Geometry: final body of the model. Coordinates: model frame, mm. Face numbers are marked on the shaded views. A direction names the side the tool comes from. Give positions to 0.01 mm unless a question says otherwise; leave off trailing zeros. Loops run counter-clockwise (first coordinate to the right, second up) from the corner with the lowest first, then second, coordinate; pieces in that order, holes last.
1. Section C-C, the plane y = 2.5. Output: boundary loops of the cut face in (x, z), then the cut area to 3 significant figures.
2. Section A-A, the plane y = -2. Output: boundary loops of the cut face in (x, z).
3. First-contact query: P1, Ø9, axis at x = -0.62, y = 5.58, coming from the -Z side; P2, Ø3, axis at x = -19, z = 0.5, coming from the +Y side; P3, Ø4, axis at x = -5, y = -2, coming from the +Z side; P4, Ø5, axis at x = -5, y = -2, coming from the -Z side. Flat tips, straight axial feed; report the tip coordinate or a pass-through.
4. Section D-D, the plane z = 3. Output: boundary loops of the cut face in (x, y) (3 decimals), then the cut area to 3 significant figures.
5. Draft query along Y for the marked faces 1, 2 and 3. Return one class per face: +Y half, -Y half, draft (parallel to the pull), parting line (faces both ways), or undercut.
6. Access query for the marked faces 4, 5 and 6. Directions: +Z, -Z, +X, -X, +Y, -Y. A direction counts if a zero-diameter tool reaches every point of the face in a straight line with its end or side. Return the directions, or none.
7. Section B-B, the plane z = -2. Output: boundary loops of the cut face in (x, y) (3 decimals), then the cut area to 3 significant figures.
8. Material intervals for line 1 along X through (y, z) = (-1, 0.5); line 2 along Y through (x, z) = (-5, 2.5); line 3 along Z through (x, y) = (0, -13.75), sorted ascending.
from build123d import *

# Parameters (mm, degrees)
SKETCH1_W                     = 46
SKETCH1_H                     = 36
BOSS_EXTRUDE1_DEPTH           = 8
M3X0_5_TAPPED_HOLE1_D         = 2.5
M3X0_5_TAPPED_HOLE1_DEPTH     = 7.5
M3X0_5_TAPPED_HOLE1_TIP       = 0.751075774
M3X0_5_TAPPED_HOLE2_D         = 2.5
M3X0_5_TAPPED_HOLE2_DEPTH     = 7.5
M3X0_5_TAPPED_HOLE2_TIP       = 0.751075774
FILLET2_R                     = 8
SKETCH13_W                    = 5
SKETCH13_H                    = 5
CUT_EXTRUDE1_DEPTH            = 4.5
CSK_FOR_M3_SFHCS1_D           = 3
CSK_FOR_M3_SFHCS1_DEPTH       = 9.5
CSK_FOR_M3_SFHCS1_CSINK_D     = 5.3
CSK_FOR_M3_SFHCS1_CSINK_ANGLE = 60
CSK_FOR_M3_SFHCS1_TIP         = 0.901290929
FILLET3_R                     = 1
HOLE1_D                       = 10
HOLE1_CBORE_D                 = 12
HOLE1_CBORE_DEPTH             = 3.3
CSK_FOR_M3_SFHCS2_D           = 3
CSK_FOR_M3_SFHCS2_DEPTH       = 9.5
CSK_FOR_M3_SFHCS2_CSINK_D     = 5.4
CSK_FOR_M3_SFHCS2_CSINK_ANGLE = 60
CSK_FOR_M3_SFHCS2_TIP         = 0.901290929


with BuildPart() as part:
    # Sketch1 → Boss-Extrude1 (new body)
    with BuildSketch(Plane.XY.offset(4.5)):
        Rectangle(SKETCH1_W, SKETCH1_H)
    extrude(amount=-BOSS_EXTRUDE1_DEPTH)

    # M3x0.5 Tapped Hole1
    with Locations(Plane(origin=(0, -18, 0), x_dir=(-1, 0, 0), z_dir=(0, -1, 0))):
        with Locations((0, -0.5)):
            Hole(M3X0_5_TAPPED_HOLE1_D / 2, depth=M3X0_5_TAPPED_HOLE1_DEPTH)
            with Locations((0, 0, -(M3X0_5_TAPPED_HOLE1_DEPTH + M3X0_5_TAPPED_HOLE1_TIP / 2))):  # 118° drill point
                Cone(0, M3X0_5_TAPPED_HOLE1_D / 2, M3X0_5_TAPPED_HOLE1_TIP, mode=Mode.SUBTRACT)

    # M3x0.5 Tapped Hole2
    with Locations(Plane(origin=(0, -18, 0), x_dir=(-1, 0, 0), z_dir=(0, -1, 0))):
        with Locations((-19, -0.5), (19, -0.5)):
            Hole(M3X0_5_TAPPED_HOLE2_D / 2, depth=M3X0_5_TAPPED_HOLE2_DEPTH)
            with Locations((0, 0, -(M3X0_5_TAPPED_HOLE2_DEPTH + M3X0_5_TAPPED_HOLE2_TIP / 2))):  # 118° drill point
                Cone(0, M3X0_5_TAPPED_HOLE2_D / 2, M3X0_5_TAPPED_HOLE2_TIP, mode=Mode.SUBTRACT)

    # Fillet2
    fillet2_edges = [part.edges().sort_by_distance(p)[0] for p in [
        (-23, 18, 0.5),
        (23, 18, 0.5),
    ]]
    fillet(fillet2_edges, radius=FILLET2_R)

    # Sketch13 → Cut-Extrude1 (cut)
    with BuildSketch(Plane.XY.offset(4.5)):
        with Locations((-5, -2)):
            Rectangle(SKETCH13_W, SKETCH13_H)
    extrude(amount=-CUT_EXTRUDE1_DEPTH, mode=Mode.SUBTRACT)

    # CSK for M3 SFHCS1
    with Locations(Plane(origin=(-5, -2, -3.5), x_dir=(-1, 0, 0), z_dir=(0, 0, -1))):
        with Locations((0, 0)):
            CounterSinkHole(CSK_FOR_M3_SFHCS1_D / 2, CSK_FOR_M3_SFHCS1_CSINK_D / 2, depth=CSK_FOR_M3_SFHCS1_DEPTH, counter_sink_angle=CSK_FOR_M3_SFHCS1_CSINK_ANGLE)
            with Locations((0, 0, -(CSK_FOR_M3_SFHCS1_DEPTH + CSK_FOR_M3_SFHCS1_TIP / 2))):  # 118° drill point
                Cone(0, CSK_FOR_M3_SFHCS1_D / 2, CSK_FOR_M3_SFHCS1_TIP, mode=Mode.SUBTRACT)

    # Fillet3
    fillet3_edges = [part.edges().sort_by_distance(p)[0] for p in [
        (-2.5, 0.5, 2.25),
        (-2.5, -4.5, 2.25),
        (-7.5, -4.5, 2.25),
        (-7.5, 0.5, 2.25),
    ]]
    fillet(fillet3_edges, radius=FILLET3_R)

    # Hole1 (through all)
    with Locations(Plane(origin=(0, 0, -3.5), x_dir=(-1, 0, 0), z_dir=(0, 0, -1))):
        with Locations((0.625, 5.577722283)):
            CounterBoreHole(HOLE1_D / 2, HOLE1_CBORE_D / 2, HOLE1_CBORE_DEPTH)

    # CSK for M3 SFHCS2
    with Locations(Plane.XY.offset(4.5)):
        with Locations((-10.337423522, 10.741909474), (8.703529058, 11.40683419), (-0.241105536, -5.415576815)):
            CounterSinkHole(CSK_FOR_M3_SFHCS2_D / 2, CSK_FOR_M3_SFHCS2_CSINK_D / 2, depth=CSK_FOR_M3_SFHCS2_DEPTH, counter_sink_angle=CSK_FOR_M3_SFHCS2_CSINK_ANGLE)
            with Locations((0, 0, -(CSK_FOR_M3_SFHCS2_DEPTH + CSK_FOR_M3_SFHCS2_TIP / 2))):  # 118° drill point
                Cone(0, CSK_FOR_M3_SFHCS2_D / 2, CSK_FOR_M3_SFHCS2_TIP, mode=Mode.SUBTRACT)


solid = part.part
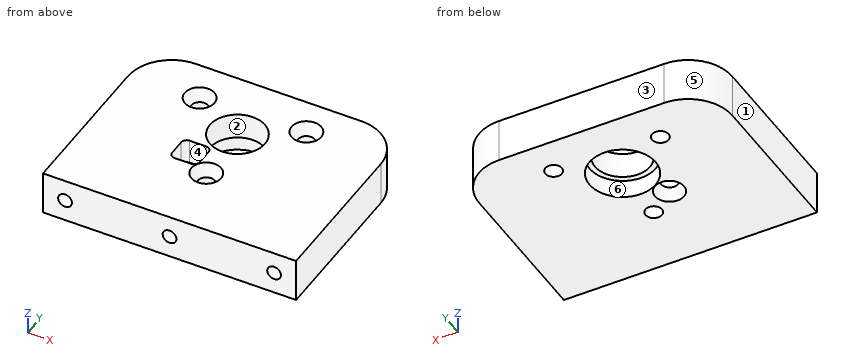
Answers below:
1. outline: (-23, -3.5) - (-5.78, -3.5) - (-5.78, -0.2) - (-4.57, -0.2) - (-4.57, 4.5) - (-23, 4.5) - close; (3.32, -0.2) - (4.53, -0.2) - (4.53, -3.5) - (23, -3.5) - (23, 4.5) - (3.32, 4.5) - close
1. area: 297 mm2
2. outline: (-23, -3.5) - (-7.65, -3.5) - (-6.5, -1.51) - (-6.5, 0) - (-7.5, 0) - (-7.5, 4.5) - (-23, 4.5) - close; (-3.5, -1.51) - (-2.35, -3.5) - (23, -3.5) - (23, 4.5) - (-2.5, 4.5) - (-2.5, 0) - (-3.5, 0) - close
3. P1: passes through
3. P2: stops at y = 17.6
3. P3: stops at z = 0
3. P4: stops at z = -3.24
4. outline: (-23, -18) - (23, -18) - (23, 10) arc R8 ccw to (15, 18) - (-15, 18) arc R8 ccw to (-23, 10) - close; hole circle Ø3.668 at (-10.337, 10.742); hole (-7.5, -3.5) arc R1 ccw to (-6.5, -4.5) - (-3.5, -4.5) arc R1 ccw to (-2.5, -3.5) - (-2.5, -0.5) arc R1 ccw to (-3.5, 0.5) - (-6.5, 0.5) arc R1 ccw to (-7.5, -0.5) - close; hole circle Ø10 at (-0.625, 5.578); hole circle Ø3.668 at (-0.241, -5.416); hole circle Ø3.668 at (8.704, 11.407)
4. area: 1,490 mm2
5. face 1: draft
5. face 2: undercut
5. face 3: +Y half
6. face 4: +Z
6. face 5: +Z, -Z, -X, +Y
6. face 6: -Z
7. outline: (-23, -18) - (23, -18) - (23, 10) arc R8 ccw to (15, 18) - (-15, 18) arc R8 ccw to (-23, 10) - close; hole circle Ø3 at (-10.337, 10.742); hole circle Ø3.568 at (-5, -2); hole circle Ø12 at (-0.625, 5.578); hole circle Ø3 at (-0.241, -5.416); hole circle Ø3 at (8.704, 11.407)
7. area: 1,480 mm2
8. line 1: x = -23 to -7.5, -2.5 to 23
8. line 2: y = -18 to -4.5, 0.5 to 3.16, 8 to 18
8. line 3: z = -3.5 to -0.75, 1.75 to 4.5
